For this review, take the finished solid that the model builds, in its own axes (mm). Face numbers are marked on the shaded views. A direction names the side the tool comes from. Round coordinates to 2 decimals unless told otherwise and drop trailing zeros. Order: outer loops, then holes, each group sorted by start corner. A loop starts at its lowest first (then second) coordinate and runs counter-clockwise, first axis right, second up. Notation, with made-up numbers: (52.5, -23.5) - (110.5, -23.5) arc R11 ccw to (110.5, -17.5) - close; hole circle Ø9 at (53, 51). An arc over 180 degrees is marked (long way). One line per item, written item: value.
```python
from build123d import *

# Parameters (mm, degrees)
SKETCH1_W           = 40
SKETCH1_H           = 40
BOSS_EXTRUDE1_DEPTH = 5
SKETCH3_R           = 13.891
CUT_EXTRUDE1_DEPTH  = 57.789083458
SKETCH4_R           = 1.664017503
BOSS_EXTRUDE3_DEPTH = 20
SKETCH5_W           = 5
SKETCH5_H           = 5
BOSS_EXTRUDE4_DEPTH = 15
SKETCH6_W           = 5
SKETCH6_H           = 5
BOSS_EXTRUDE5_DEPTH = 100
SKETCH7_R           = 15.460977434
SKETCH7_R_2         = 13.828216596
BOSS_EXTRUDE6_DEPTH = 5
SKETCH8_W           = 11.277313534
SKETCH8_H           = 8.274115908
BOSS_EXTRUDE7_DEPTH = 5
FILLET1_R           = 4
FILLET2_R           = 4


with BuildPart() as part:
    # Sketch1 → Boss-Extrude1 (new body)
    with BuildSketch(Plane.XY):
        with Locations((20, -20)):
            Rectangle(SKETCH1_W, SKETCH1_H)
    boss_extrude1 = extrude(amount=BOSS_EXTRUDE1_DEPTH)

    # Sketch3 → Cut-Extrude1 (cut, through all)
    with BuildSketch(Plane(origin=(0, 0, 0), x_dir=(-1, 0, 0), z_dir=(0, 0, -1))):
        with Locations((-20, -20)):
            Circle(SKETCH3_R)
    extrude(amount=-CUT_EXTRUDE1_DEPTH, mode=Mode.SUBTRACT)

    # Sketch4 → Boss-Extrude3 (add)
    with BuildSketch(Plane.XY.offset(5)):
        with Locations((4, -4)):
            Circle(SKETCH4_R)
        with Locations((36, -4)):
            Circle(SKETCH4_R)
        with Locations((36, -36)):
            Circle(SKETCH4_R)
        with Locations((4, -36)):
            Circle(SKETCH4_R)
    extrude(amount=BOSS_EXTRUDE3_DEPTH)

    # Mirror1: Boss-Extrude1 across plane
    add(boss_extrude1.mirror(Plane.XY.offset(15)))

    # Sketch5 → Boss-Extrude4 (add)
    with BuildSketch(Plane.XY.offset(30)):
        with Locations((20, -20)):
            Rectangle(SKETCH5_W, SKETCH5_H)
    extrude(amount=BOSS_EXTRUDE4_DEPTH)

    # Sketch6 → Boss-Extrude5 (add)
    with BuildSketch(Plane.XZ.offset(22.5)):
        with Locations((20, 42.5)):
            Rectangle(SKETCH6_W, SKETCH6_H)
    extrude(amount=BOSS_EXTRUDE5_DEPTH)

    # Sketch7 → Boss-Extrude6 (add)
    with BuildSketch(Plane(origin=(0, 0, 0), x_dir=(-1, 0, 0), z_dir=(0, 0, -1))):
        with Locations(Location((-20, -20, 0), (0, 0, 180))):
            Circle(SKETCH7_R)
        with Locations((-20, -20)):
            Circle(SKETCH7_R_2, mode=Mode.SUBTRACT)
    boss_extrude6 = extrude(amount=BOSS_EXTRUDE6_DEPTH)

    # Mirror3: Boss-Extrude6 across plane
    add(boss_extrude6.mirror(Plane.XY.offset(2.5)))

    # Sketch8 → Boss-Extrude7 (add)
    with BuildSketch(Plane.XZ.offset(122.5)):
        with Locations((19.966542914, 42.419592184)):
            Rectangle(SKETCH8_W, SKETCH8_H)
    extrude(amount=BOSS_EXTRUDE7_DEPTH)

    # Fillet1
    fillet1_edges = [part.edges().sort_by_distance(p)[0] for p in [
        (0, 0, 2.5),
    ]]
    fillet(fillet1_edges, radius=FILLET1_R)

    # Fillet2
    fillet2_edges = [part.edges().sort_by_distance(p)[0] for p in [
        (0, -40, 27.5),
        (0, 0, 27.5),
        (40, 0, 27.5),
        (40, -40, 27.5),
        (40, 0, 2.5),
        (40, -40, 2.5),
        (0, -40, 2.5),
    ]]
    fillet(fillet2_edges, radius=FILLET2_R)


solid = part.part
```
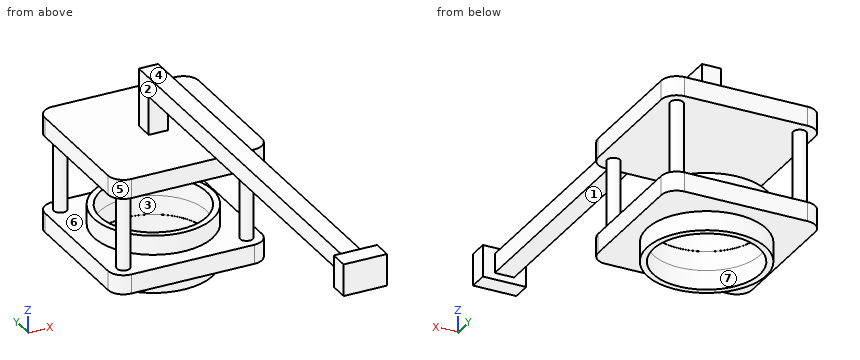
Item 1: Take a section at A-A (y = -20). Count the separate pieces of the cut face and the enclosed holes in it, plus the area to 3 significant figures.
Returned:
separate pieces: 3
enclosed holes: 0
area: 369 mm^2
Item 2: For P1, Ø4, axis at y = -126, z = 42, coming from the -X side; P2, Ø10, axis at x = 15, z = 14.5, coming from the +Y side; P3, Ø16.5, axis at x = 20, y = -20, coming from the -Z side, all flat-tipped, find the tip position at first contact; note any pin that passes through.
Returned:
P1: x = 14.33
P2: y = -4.8
P3: z = 25
Item 3: Machinability: for the marked faces 4, 5, 6 and 7, which of the approach directions +Z, -Z, +X, -X, +Y, -Y give a long, thin tool a straight path to every point of the face, cutting with its end or side? Answer none if there is none.
Returned:
face 4: +Z, +X, -X, +Y
face 5: +Z, -Z, -X, -Y
face 6: none
face 7: -Z
Item 4: Take a section at C-C (z = 42.5). Write out the cut boundary in (x, y), plus the area to 3 significant figures.
Returned:
outline: (14.33, -127.5) - (25.61, -127.5) - (25.61, -122.5) - (22.5, -122.5) - (22.5, -17.5) - (17.5, -17.5) - (17.5, -122.5) - (14.33, -122.5) - close
area: 581 mm^2
Item 5: Wall thickness on line 1 (Z direction, x = 12.5, y = -6); line 2 (Z direction, x = 20, y = -32); line 3 (Y direction, x = 20, z = 2.15): over which ranges is each line inside the solid? List them lowest first.
Returned:
line 1: 0 to 5, 25 to 30
line 2: 25 to 30, 40 to 45
line 3: -40 to -33.89, -6.11 to 0
Item 6: Take a section at D-D (z = 20.5). Write out the cut boundary in (x, y), plus the area to 3 significant figures.
Returned:
outline: circle Ø3.33 at (4, -36); circle Ø3.33 at (4, -4); circle Ø3.33 at (36, -36); circle Ø3.33 at (36, -4)
area: 34.8 mm^2
Item 7: The part is to be moulded in two halves that separate along X. For the marked faces 1, 2 and 3, say which applies: +X half, -X half, draft (parallel to the pull), parting line (faces both ways), or undercut.
Returned:
face 1: draft
face 2: -X half
face 3: undercut
Item 8: Take a section at B-B (x = 10). Write out the cut boundary in (y, z), plus the area to 3 significant figures.
Returned:
outline: (-40, 0) - (-31.79, 0) - (-31.79, -5) - (-29.55, -5) - (-29.55, 0) - (-29.64, 0) - (-29.64, 5) - (-29.55, 5) - (-29.55, 10) - (-31.79, 10) - (-31.79, 5) - (-40, 5) - close; (-40, 25) - (0, 25) - (0, 30) - (-40, 30) - close; (-10.45, -5) - (-8.21, -5) - (-8.21, 0) - (0, 0) - (0, 5) - (-8.21, 5) - (-8.21, 10) - (-10.45, 10) - (-10.45, 5) - (-10.36, 5) - (-10.36, 0) - (-10.45, 0) - close
area: 348 mm^2
